```python
from build123d import *

# Parameters (mm, degrees)
SKETCH1_W           = 81.28
SKETCH1_H           = 81.28
BOSS_EXTRUDE1_DEPTH = 88.9
SHELL1_T            = -2.54
SKETCH4_W           = 78.74
SKETCH4_H           = 78.74
CUT_EXTRUDE2_DEPTH  = 5.08
CUT_EXTRUDE3_DEPTH  = 17.78


with BuildPart() as part:
    # Sketch1 → Boss-Extrude1 (new body)
    with BuildSketch(Plane.XY):
        Rectangle(SKETCH1_W, SKETCH1_H)
    extrude(amount=BOSS_EXTRUDE1_DEPTH)

    # Shell1
    shell1_openings = [part.faces().sort_by_distance(p)[0] for p in [
        (0, 0, 0),
    ]]
    offset(amount=SHELL1_T, openings=shell1_openings, kind=Kind.INTERSECTION)

    # Sketch4 → Cut-Extrude2 (cut)
    with BuildSketch(Plane(origin=(0, 0, 0), x_dir=(-1, 0, 0), z_dir=(0, 0, -1))):
        Rectangle(SKETCH4_W, SKETCH4_H)
    extrude(amount=-CUT_EXTRUDE2_DEPTH, mode=Mode.SUBTRACT)

    # Sketch5 → Cut-Extrude3 (cut)
    with BuildSketch(Plane.XY.offset(88.9)):
        with BuildLine():
            Line((-36.729338969, 32.846931931), (-36.729338969, 21.496884439))
            ThreePointArc((-36.729338969, 21.496884439), (-35.161354887, 19.150230426), (-32.393287744, 19.700833215))
            Line((-32.393287744, 19.700833215), (-21.043240252, 31.050880707))
            ThreePointArc((-21.043240252, 31.050880707), (-20.492637463, 33.81894785), (-22.839291476, 35.386931931))
            Line((-22.839291476, 35.386931931), (-34.189338969, 35.386931931))
            ThreePointArc((-34.189338969, 35.386931931), (-35.985390193, 34.642983156), (-36.729338969, 32.846931931))
        make_face()
        with BuildLine():
            Line((32.393287744, 19.700833215), (21.043240252, 31.050880707))
            ThreePointArc((21.043240252, 31.050880707), (20.492637463, 33.81894785), (22.839291476, 35.386931931))
            Line((22.839291476, 35.386931931), (34.189338969, 35.386931931))
            ThreePointArc((34.189338969, 35.386931931), (35.985390193, 34.642983156), (36.729338969, 32.846931931))
            Line((36.729338969, 32.846931931), (36.729338969, 21.496884439))
            ThreePointArc((36.729338969, 21.496884439), (35.161354887, 19.150230426), (32.393287744, 19.700833215))
        make_face()
        with BuildLine():
            Line((32.393287744, -19.700833215), (21.043240252, -31.050880707))
            ThreePointArc((21.043240252, -31.050880707), (20.492637463, -33.81894785), (22.839291476, -35.386931931))
            Line((22.839291476, -35.386931931), (34.189338969, -35.386931931))
            ThreePointArc((34.189338969, -35.386931931), (35.985390193, -34.642983156), (36.729338969, -32.846931931))
            Line((36.729338969, -32.846931931), (36.729338969, -21.496884439))
            ThreePointArc((36.729338969, -21.496884439), (35.161354887, -19.150230426), (32.393287744, -19.700833215))
        make_face()
        with BuildLine():
            Line((-32.393287744, -19.700833215), (-21.043240252, -31.050880707))
            ThreePointArc((-21.043240252, -31.050880707), (-20.492637463, -33.81894785), (-22.839291476, -35.386931931))
            Line((-22.839291476, -35.386931931), (-34.189338969, -35.386931931))
            ThreePointArc((-34.189338969, -35.386931931), (-35.985390193, -34.642983156), (-36.729338969, -32.846931931))
            Line((-36.729338969, -32.846931931), (-36.729338969, -21.496884439))
            ThreePointArc((-36.729338969, -21.496884439), (-35.161354887, -19.150230426), (-32.393287744, -19.700833215))
        make_face()
    extrude(amount=-CUT_EXTRUDE3_DEPTH, mode=Mode.SUBTRACT)


solid = part.part
```
The listing builds one solid part. Answer for the finished solid, in the listing's coordinates (mm). A direction names the side the tool comes from. Give positions to 0.01 mm unless a question says otherwise; leave off trailing zeros. Order: outer loops, then holes, each group sorted by start corner. A loop starts at its lowest first (then second) coordinate and runs counter-clockwise, first axis right, second up. Notation, with made-up numbers: M 61,50 L 85,50 A25 cw 85,68 Z; hole C 87.25,75 d7. An arc over 180 degrees is marked long. Put each result on its own line as item: value. Start each with the question number.
Item 1: A flat-ended cylindrical pin translates along its axis: P1, Ø8, axis at x = -11, y = -19.5, coming from the -Z side. Find the tip coordinate at first contact, or state that the pin passes through.
Item 2: The part is cut by section C-C, the plane z = 33.5. Determine the outline of the cut face in (x, y), and give its area (3 significant figures).
Item 3: Which of the six approach directions +Z, -Z, +X, -X, +Y, -Y give full straight-line access (tool end or side, diameter ignored) to faces 1 (the face through (40.64, -1, 44)), 2 (the face through (-28, -35.387, 88)), 3 (the face through (-39.37, -1, 3))?
Item 4: Find the intervals of material crossed by line 1 along Y through (x, z) = (-13, 72); line 2 along Z through (x, y) = (18, 30.5), in increasing order.
Item 5: For a pull along Y with two mould halves and no side action, classify faces 4 (the face through (38.1, -1, 45)), 5 (the face through (-36.729, -27, 88)), 6 (the face through (-40.64, -1, 44)), 7 (the face through (-1, -40.64, 44)) as +Y half, -Y half, draft (parallel to the pull), parting line (faces both ways), or undercut.
Item 6: The part is cut by section D-D, the plane x = -31. Determine the outline of the cut face in (y, z), and give its area (3 significant figures).
Item 7: The part is cut by section A-A, the plane x = 6. Determine the outline of the cut face in (y, z).
Answer key:
1. P1: stops at z = 86.36
2. outline: M -40.64,-40.64 L 40.64,-40.64 L 40.64,40.64 L -40.64,40.64 Z; hole M -38.1,-38.1 L 38.1,-38.1 L 38.1,38.1 L -38.1,38.1 Z
2. area: 800 mm²
3. face 1: +Z, -Z, +X, +Y, -Y
3. face 2: +Z, -Z
3. face 3: -Z
4. line 1: y = -40.64 to -38.1, 38.1 to 40.64
4. line 2: z = 86.36 to 88.9
5. face 4: undercut
5. face 5: undercut
5. face 6: draft
5. face 7: -Y half
6. outline: M -40.64,0 L -39.37,0 L -39.37,5.08 L -38.1,5.08 L -38.1,86.36 L -35.39,86.36 L -35.39,88.9 L -40.64,88.9 Z; M -21.09,86.36 L 21.09,86.36 L 21.09,88.9 L -21.09,88.9 Z; M 35.39,86.36 L 38.1,86.36 L 38.1,5.08 L 39.37,5.08 L 39.37,0 L 40.64,0 L 40.64,88.9 L 35.39,88.9 Z
6. area: 560 mm²
7. outline: M -40.64,0 L -39.37,0 L -39.37,5.08 L -38.1,5.08 L -38.1,86.36 L 38.1,86.36 L 38.1,5.08 L 39.37,5.08 L 39.37,0 L 40.64,0 L 40.64,88.9 L -40.64,88.9 Z
